Design review of the part built by this model. Coordinates are the model's own, in mm. A direction names the side the tool comes from. Coordinates: 2 decimals unless noted, no trailing zeros. Order: outer loops, then holes, each group sorted by start corner. A loop starts at its lowest first (then second) coordinate and runs counter-clockwise, first axis right, second up. Notation, with made-up numbers: (40, 83) - (49, 83) arc R28 ccw to (49, 111) - close; hole circle Ø10 at (23, 1.5). An arc over 180 degrees is marked (long way). Write each question's results on one line, items separated by ' | '. Start each with the question number.
```python
from build123d import *

# Parameters (mm, degrees)
SKETCH1_R           = 8
SKETCH1_W           = 5.5
SKETCH1_H           = 3.7
BOSS_EXTRUDE1_DEPTH = 5
CUT_EXTRUDE1_DEPTH  = 13.369316877
CIRPATTERN1_COUNT   = 6


with BuildPart() as part:
    # Sketch1 → Boss-Extrude1 (new body)
    with BuildSketch(Plane.XY):
        Circle(SKETCH1_R)
        Rectangle(SKETCH1_W, SKETCH1_H, mode=Mode.SUBTRACT)
    extrude(amount=BOSS_EXTRUDE1_DEPTH)

    # Sketch2 → Cut-Extrude1 (cut, through all)
    with BuildSketch(Plane.XY):
        Polygon((-7.331932906, 22.221764399), (0, 24.952212466), (7.331932906, 22.221764399), (3.798424573, 7.040736522), (3.120998591, 6.924019842), (1.330058439, 5.723612136), (0.501497444, 4.50257488), (-0.501497444, 4.50257488), (-1.330058439, 5.723612136), (-3.120998591, 6.924019842), (-3.798424573, 7.040736522), align=None)
    cut_extrude1 = extrude(amount=CUT_EXTRUDE1_DEPTH, mode=Mode.SUBTRACT)

    # CirPattern1: Cut-Extrude1 ×6 about axis
    cirpattern1_axis = Axis((0, 0, 0), (0, 0, 1))
    for i in range(1, CIRPATTERN1_COUNT):
        add(cut_extrude1.rotate(cirpattern1_axis, i * 360 / CIRPATTERN1_COUNT), mode=Mode.SUBTRACT)


solid = part.part
```
(1) Take a section at D-D (y = 3.25). State the section outline as (x, z) points, plus the area to 3 significant figures.
(2) Take a section at C-C (y = -3.75). State the section outline as (x, z) points.
(3) Take a section at A-A (x = 0.25). State the section outline as (y, z) points, plus the area to 3 significant figures.
(4) Clearance check with flat-ended pins moving along their axes: pin 1 (3 mm diameter, centred on y = 3, z = 4, fed in from -X); pin 2 (1.5 mm diameter, centred on x = -0.5, z = 3.5, fed in from +Y). State where each tip first meets the part, or that it passes through.
(5) Take a section at B-B (y = 1.5). State the section outline as (x, z) points, plus the area to 3 significant figures.
(6) Tool access review of faces 5 (the face through (0.91, -5.105, 2.465)), 6 (the face through (-3.9, -2.25, 2.46)), 7 (the face through (4.896, 1.763, 2.465)), 8 (the face through (-6.6, -1.23, 2.46)), 9 (the face through (2.238, 6.332, 2.465)): name each direction out of +Z, -Z, +X, -X, +Y, -Y from which nothing blocks a thin tool from reaching the whole face with its end or side.
(7) To check wall thickness, follow line 1 along Y through (x, z) = (0, 3.25); line 2 along Y through (x, z) = (4, 2.85); line 3 along Y through (x, z) = (3.75, 0.9). State the ranges of each line that lie inside material, in increasing order. Write a range as [from, to].
(8) Mouldability with a two-part tool opening along Y and no side actions: class faces 1 (the face through (6.58, -1.24, 2.46)), 2 (the face through (0, -3, 5)), 3 (the face through (4.876, -1.764, 2.465)), 4 (the face through (6.6, 1.23, 2.46)) as +Y half, -Y half, draft (parallel to the pull), parting line (faces both ways), or undercut.
Worked out:
1) outline: (-3.92, 0) - (3.92, 0) - (3.92, 5) - (-3.92, 5) - close | area: 39.2 mm^2
2) outline: (-4.16, 0) - (4.16, 0) - (4.16, 5) - (-4.16, 5) - close
3) outline: (-4.5, 0) - (-1.85, 0) - (-1.85, 5) - (-4.5, 5) - close; (1.85, 0) - (4.5, 0) - (4.5, 5) - (1.85, 5) - close | area: 26.5 mm^2
4) pin 1: x = -6.05 | pin 2: y = 5.61
5) outline: (-6.05, 0) - (-2.75, 0) - (-2.75, 5) - (-6.05, 5) - close; (2.75, 0) - (6.05, 0) - (6.05, 5) - (2.75, 5) - close | area: 33.0 mm^2
6) face 5: +Z, -Z, -Y | face 6: +Z, -Z, -X | face 7: +Z, -Z, +X | face 8: +Z, -Z, -X, -Y | face 9: +Z, -Z, +Y
7) line 1: [-4.5, -1.85], [1.85, 4.5] | line 2: [-6.93, -3.41], [-2.08, 2.08], [3.41, 6.93] | line 3: [-7.03, -2.89], [-2.51, 2.51], [2.89, 7.03]
8) face 1: -Y half | face 2: draft | face 3: undercut | face 4: +Y half
